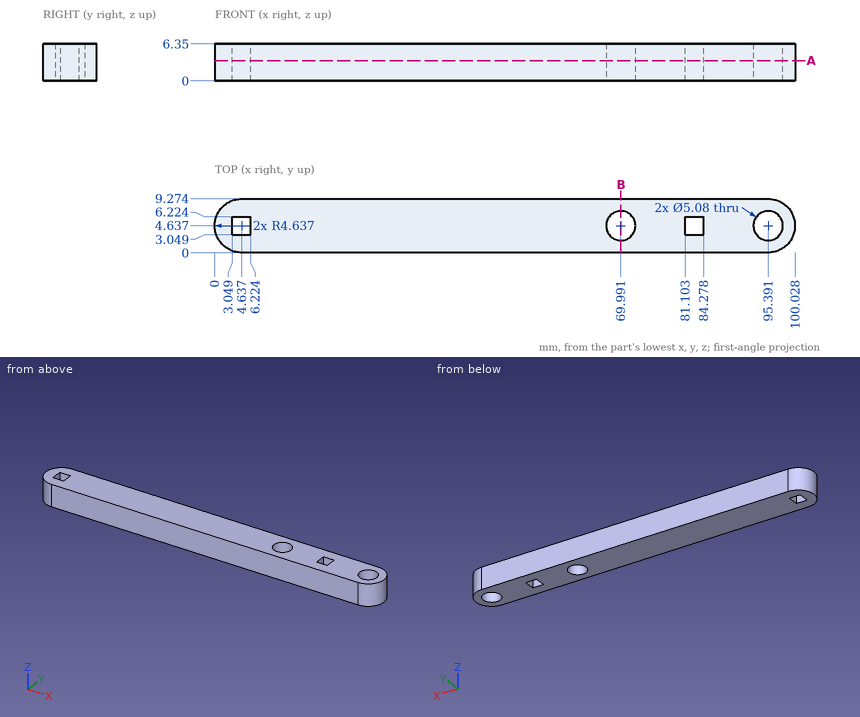
Can you work these out from the drawing? Everything is in mm from the part's minimum corner. Round coordinates to 2 decimals unless told otherwise and drop trailing zeros. Write each loop counter-clockwise with the first axis right and the second up, starting at its lowest first coordinate (ties: lowest second). Pieces come first, ordered by that corner, then holes. Notation, with made-up numbers: (28, 12.25) - (58, 12.25) arc R14 cw to (58, 16.25) - close; hole circle Ø10 at (25.5, 35.5). An arc over 180 degrees is marked (long way). Write each question's results on one line, items separated by ' | '. Start each with the question number.
1) Suppose I cut it at A-A (z = 3.5). Give the number of separate pieces and of enclosed holes in the cut face.
2) For pin 1 Ø3 at (y, z) = (2.5, 5.5) entering from -X; pin 2 Ø4.5 at (x, y) = (95.39, 4.64) entering from -Z; pin 3 Ø1.5 at (y, z) = (1, 1) entering from -X; pin 4 Ø1 at (y, z) = (4, 3) entering from +X, each with a flat end and sliding along its axis, tell me the tip position at first contact or that it passes through.
3) Please list where these lines run through material, in increasing order: line 1 (X direction, y = 2.75, z = 3.25) (1 decimal); line 2 (Y direction, x = 71.5, z = 4.75) (1 decimal); line 3 (X direction, y = 0.5, z = 5) (1 decimal).
4) Suppose I cut it at B-B (x = 70). List the corners of the cut face in (y, z) for me.
Here are the results:
1) separate pieces: 1 | enclosed holes: 4
2) pin 1: stops at x = 0.04 | pin 2: passes through | pin 3: stops at x = 1.01 | pin 4: stops at x = 100.03
3) line 1: x = 0.4 to 68.3, 71.7 to 93.7, 97.1 to 99.6 | line 2: y = 0 to 2.6, 6.7 to 9.3 | line 3: x = 2.5 to 97.5
4) outline: (0, 0) - (2.1, 0) - (2.1, 6.35) - (0, 6.35) - close; (7.18, 0) - (9.27, 0) - (9.27, 6.35) - (7.18, 6.35) - close
